Can you work these out from the model? Positions are in its coordinate system, mm. Face numbers are marked on the shaded views. A direction names the side the tool comes from. Give positions to 0.01 mm unless a question says otherwise; leave off trailing zeros. Loops run counter-clockwise (first coordinate to the right, second up) from the corner with the lowest first, then second, coordinate; pieces in that order, holes last. Notation, with made-up numbers: (30.5, -15.75) - (78.5, -15.75) arc R14 cw to (78.5, 2.25) - close; hole circle Ø10 at (4.25, 16). An arc over 180 degrees is marked (long way). Answer as a JSON object with one key per item and string values.
```python
from build123d import *

# Parameters (mm, degrees)
ESQUISSE2_W             = 1036
ESQUISSE2_H             = 650
BOSS_EXTRU_1_DEPTH      = 20
ESQUISSE3_W             = 620
ESQUISSE3_H             = 620
ENL_V_MAT_EXTRU_1_DEPTH = 10
ESQUISSE4_W             = 600
ESQUISSE4_H             = 600
ENL_V_MAT_EXTRU_2_DEPTH = 10
ESQUISSE5_W             = 50
ESQUISSE5_H             = 50
BOSS_EXTRU_2_DEPTH      = 780
ESQUISSE6_W             = 16
ESQUISSE6_H             = 550
BOSS_EXTRU_3_DEPTH      = 620
BOSS_EXTRU_5_DEPTH      = 20
ESQUISSE10_W            = 150
ESQUISSE10_H            = 400
BOSS_EXTRU_6_DEPTH      = 175
ESQUISSE20_R            = 25
ENL_V_MAT_EXTRU_4_DEPTH = 16
ESQUISSE21_W            = 936
ESQUISSE21_H            = 620
BOSS_EXTRU_7_DEPTH      = 16
BOSS_EXTRU_8_DEPTH      = 618
ESQUISSE25_W            = 200
ESQUISSE25_H            = 575
ENL_V_MAT_EXTRU_5_DEPTH = 16
ESQUISSE26_W            = 16
ESQUISSE26_H            = 575
BOSS_EXTRU_9_DEPTH      = 200


with BuildPart() as part:
    # Esquisse2 → Boss.-Extru.1 (new body)
    with BuildSketch(Plane(origin=(0, 0, 0), x_dir=(1, 0, 0), z_dir=(0, 1, 0))):
        with Locations((476.22027439, -276.413871951)):
            Rectangle(ESQUISSE2_W, ESQUISSE2_H)
    extrude(amount=BOSS_EXTRU_1_DEPTH)

    # Esquisse3 → Enlèv. mat.-Extru.1 (cut)
    with BuildSketch(Plane(origin=(0, 20, 0), x_dir=(1, 0, 0), z_dir=(0, 1, 0))):
        with Locations((544.22027439, -276.413871951)):
            Rectangle(ESQUISSE3_W, ESQUISSE3_H)
    extrude(amount=-ENL_V_MAT_EXTRU_1_DEPTH, mode=Mode.SUBTRACT)

    # Esquisse4 → Enlèv. mat.-Extru.2 (cut)
    with BuildSketch(Plane(origin=(0, 10, 0), x_dir=(1, 0, 0), z_dir=(0, 1, 0))):
        with Locations((544.22027439, -276.413871951)):
            Rectangle(ESQUISSE4_W, ESQUISSE4_H)
    extrude(amount=-ENL_V_MAT_EXTRU_2_DEPTH, mode=Mode.SUBTRACT)

    # Esquisse5 → Boss.-Extru.2 (add)
    with BuildSketch(Plane.XZ):
        with Locations((-16.77972561, 576.413871951)):
            Rectangle(ESQUISSE5_W, ESQUISSE5_H)
        with Locations((969.22027439, 576.413871951)):
            Rectangle(ESQUISSE5_W, ESQUISSE5_H)
        with Locations((-16.77972561, -23.586128049)):
            Rectangle(ESQUISSE5_W, ESQUISSE5_H)
        with Locations((969.22027439, -23.586128049)):
            Rectangle(ESQUISSE5_W, ESQUISSE5_H)
    extrude(amount=BOSS_EXTRU_2_DEPTH)

    # Esquisse6 → Boss.-Extru.3 (add)
    with BuildSketch(Plane.XZ):
        with Locations((-33.77972561, 276.413871951)):
            Rectangle(ESQUISSE6_W, ESQUISSE6_H)
    extrude(amount=BOSS_EXTRU_3_DEPTH)

    # Esquisse8 → Boss.-Extru.5 (add)
    with BuildSketch(Plane.XZ.offset(620)):
        Polygon((-25.77972561, 551.413871951), (8.22027439, 551.413871951), (8.22027439, 585.413871951), (258.22027439, 585.413871951), (258.22027439, -32.586128049), (8.22027439, -32.586128049), (8.22027439, 1.413871951), (-25.77972561, 1.413871951), align=None)
    extrude(amount=-BOSS_EXTRU_5_DEPTH)

    # Esquisse10 → Boss.-Extru.6 (add)
    with BuildSketch(Plane(origin=(0, -600, 0), x_dir=(1, 0, 0), z_dir=(0, 1, 0))):
        with Locations((49.22027439, -276.413871951)):
            Rectangle(ESQUISSE10_W, ESQUISSE10_H)
    extrude(amount=BOSS_EXTRU_6_DEPTH)

    # Esquisse20 → Enlèv. mat.-Extru.4 (cut)
    with BuildSketch(Plane.ZY.offset(41.77972561)):
        with Locations((31.413871951, -30)):
            Circle(ESQUISSE20_R)
    extrude(amount=-ENL_V_MAT_EXTRU_4_DEPTH, mode=Mode.SUBTRACT)

    # Esquisse21 → Boss.-Extru.7 (add)
    with BuildSketch(Plane(origin=(0, 0, -32.586128049), x_dir=(-1, 0, 0), z_dir=(0, 0, -1))):
        with Locations((-476.22027439, -310)):
            Rectangle(ESQUISSE21_W, ESQUISSE21_H)
    extrude(amount=BOSS_EXTRU_7_DEPTH)

    # Esquisse24 → Boss.-Extru.8 (add)
    with BuildSketch(Plane.XY.offset(-32.586128049)):
        Polygon((258.22027439, -620), (258.22027439, -600), (844.22027439, 0), (864.22027439, 0), align=None)
    extrude(amount=BOSS_EXTRU_8_DEPTH)

    # Esquisse25 → Enlèv. mat.-Extru.5 (cut)
    with BuildSketch(Plane.XY.offset(-32.586128049)):
        with Locations((123.22027439, -287.5)):
            Rectangle(ESQUISSE25_W, ESQUISSE25_H)
    extrude(amount=-ENL_V_MAT_EXTRU_5_DEPTH, mode=Mode.SUBTRACT)

    # Esquisse26 → Boss.-Extru.9 (add)
    with BuildSketch(Plane(origin=(0, 0, -48.586128049), x_dir=(-1, 0, 0), z_dir=(0, 0, -1))):
        with Locations((-15.22027439, -287.5)):
            Rectangle(ESQUISSE26_W, ESQUISSE26_H)
    extrude(amount=BOSS_EXTRU_9_DEPTH)


solid = part.part
```
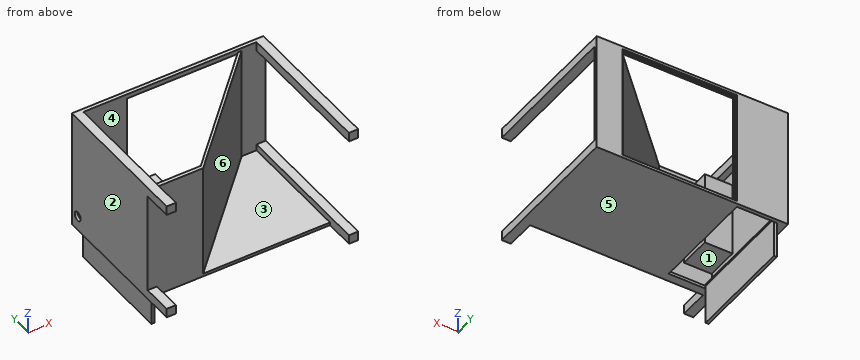
1) Imagine slicing it at D-D on y = -294. Write out the boundary of the cut face in (x, z).
Check sheet entries:
{"outline": "(-41.78, -48.59) - (7.22, -48.59) - (7.22, -248.59) - (23.22, -248.59) - (23.22, -32.59) - (8.22, -32.59) - (8.22, 1.41) - (-25.78, 1.41) - (-25.78, 551.41) - (8.22, 551.41) - (8.22, 601.41) - (-41.78, 601.41) - close; (223.22, -48.59) - (994.22, -48.59) - (994.22, 1.41) - (944.22, 1.41) - (944.22, -32.59) - (576.86, -32.59) - (576.86, 585.41) - (557.08, 585.41) - (557.08, -32.59) - (223.22, -32.59) - close; (944.22, 551.41) - (994.22, 551.41) - (994.22, 601.41) - (944.22, 601.41) - close"}
2) I'm going to push flat-ended pins straight in: P1, Ø17.5, axis at x = 16, z = -186.5, coming from the +Y side; P2, Ø6, axis at x = 451.5, z = 435, coming from the -Y side; P3, Ø2, axis at x = 674.5, z = 372.5, coming from the -Y side. Where does each tip first touch, or does it pass through?
Check sheet entries:
{"P1": "y = 0", "P2": "y = -425.32", "P3": "y = -195.13"}
3) Which directions (+Z, -Z, +X, -X, +Y, -Y) give clear straight access to the entire face, cutting with the end or side of a thin tool? Please do the marked faces 1, 2 and 3.
Check sheet entries:
{"face 1": "none", "face 2": "+Z, -Z, -X, +Y, -Y", "face 3": "+Z, -Y"}
4) I need wall thicknesses on L1, parallel to Z at x = 20, y = -499; L2, parallel to Y at x = 117, z = 472; L3, parallel to Z at x = 645, y = -149.5. Which ranges of each line are inside material? Lowest first, please.
Check sheet entries:
{"L1": "-248.59 to -32.59, 76.41 to 476.41", "L2": "-620 to -425, 0 to 20", "L3": "-48.59 to -32.59"}
5) Imagine slicing it at C-C on z = 337. Write out the boundary of the cut face in (x, y), and give its area (3 significant figures).
Check sheet entries:
{"outline": "(-41.78, -620) - (258.22, -620) - (864.22, 0) - (994.22, 0) - (994.22, 20) - (854.22, 20) - (854.22, 10) - (844.22, 10) - (844.22, 0) - (258.22, -600) - (124.22, -600) - (124.22, -425) - (-25.78, -425) - (-25.78, 0) - (244.22, 0) - (244.22, 10) - (234.22, 10) - (234.22, 20) - (-41.78, 20) - close", "area": "62,400 mm2"}
6) Imagine slicing it at A-A on y = -656.5. Write out the boundary of the cut face in (x, z).
Check sheet entries:
{"outline": "(-41.78, -48.59) - (8.22, -48.59) - (8.22, 1.41) - (-41.78, 1.41) - close; (-41.78, 551.41) - (8.22, 551.41) - (8.22, 601.41) - (-41.78, 601.41) - close; (944.22, -48.59) - (994.22, -48.59) - (994.22, 1.41) - (944.22, 1.41) - close; (944.22, 551.41) - (994.22, 551.41) - (994.22, 601.41) - (944.22, 601.41) - close"}
7) Imagine slicing it at B-B on x = 490. Write out the boundary of the cut face in (y, z).
Check sheet entries:
{"outline": "(-620, -48.59) - (20, -48.59) - (20, -33.59) - (10, -33.59) - (10, -23.59) - (0, -23.59) - (0, -32.59) - (-362.68, -32.59) - (-362.68, 585.41) - (-382.87, 585.41) - (-382.87, -32.59) - (-620, -32.59) - close; (0, 576.41) - (10, 576.41) - (10, 586.41) - (20, 586.41) - (20, 601.41) - (0, 601.41) - close"}
8) If we mould it in two halves opening along Y, with no side actions, what happens to the marked faces 4, 5 and 6? For each: released by +Y, released by -Y, zero draft, split by the parting line, or undercut.
Check sheet entries:
{"face 4": "undercut", "face 5": "zero draft", "face 6": "released by -Y"}
